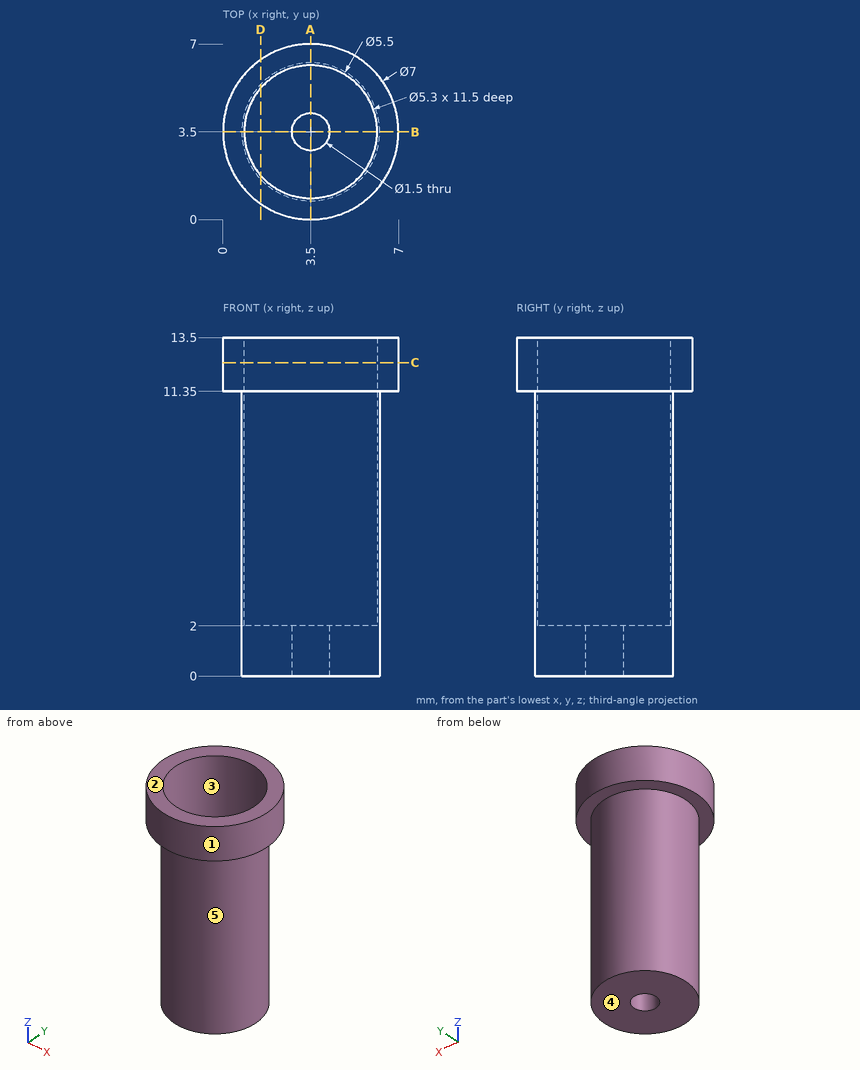
Could you check a few things on this drawing? It's one solid part, dimensions in mm from its lowest x, y, z. A direction names the side the tool comes from. Coordinates: 2 decimals unless noted, no trailing zeros. Order: outer loops, then holes, each group sorted by start corner. A loop starts at its lowest first (then second) coordinate and runs counter-clockwise, first axis right, second up. Notation, with made-up numbers: (67.25, -38.75) -> (104.25, -38.75) arc R23 ccw to (104.25, -10.75) -> close; hole circle Ø4 at (89, -27.5). An arc over 180 degrees is marked (long way). One line per item, written item: value. Start each with the question number.
1) We'd pull the mould along Y, two halves only. Please class the marked faces 1, 2 and 3: +Y half, -Y half, draft (parallel to the pull), parting line (faces both ways), or undercut.
2) Imagine slicing it at A-A on x = 3.5. List the corners of the cut face in (y, z) for me.
3) Imagine slicing it at D-D on x = 1.5. List the corners of the cut face in (y, z) for me, plus the area to 3 significant figures.
4) Imagine slicing it at C-C on z = 12.5. List the corners of the cut face in (x, y) for me, plus the area to 3 significant figures.
5) Which directions (+Z, -Z, +X, -X, +Y, -Y) give clear straight access to the entire face, cutting with the end or side of a thin tool? Please do the marked faces 4 and 5.
6) If I drill on L1, parallel to Y at x = 3.5, z = 1.35; L2, parallel to Z at x = 0.5, y = 5.25; L3, parallel to Z at x = 2.5, y = 1.25, over which ranges is the centre line in solid material (lowest first)? Write a range as [from, to].
Answer list:
1. face 1: parting line
1. face 2: draft
1. face 3: undercut
2. outline: (0, 11.35) -> (0.75, 11.35) -> (0.75, 0) -> (2.75, 0) -> (2.75, 2) -> (0.85, 2) -> (0.85, 13.5) -> (0, 13.5) -> close; (4.25, 0) -> (6.25, 0) -> (6.25, 11.35) -> (7, 11.35) -> (7, 13.5) -> (6.15, 13.5) -> (6.15, 2) -> (4.25, 2) -> close
3. outline: (0.63, 11.35) -> (1.61, 11.35) -> (1.61, 0) -> (5.39, 0) -> (5.39, 11.35) -> (6.37, 11.35) -> (6.37, 13.5) -> (5.24, 13.5) -> (5.24, 2) -> (1.76, 2) -> (1.76, 13.5) -> (0.63, 13.5) -> close
3. area: 15.2 mm2
4. outline: circle Ø7 at (3.5, 3.5); hole circle Ø5.3 at (3.5, 3.5)
4. area: 16.4 mm2
5. face 4: -Z, +X, -X, +Y, -Y
5. face 5: -Z
6. L1: y = [0.75, 2.75], [4.25, 6.25]
6. L2: z = [11.35, 13.5]
6. L3: z = [0, 2]
